The model under review builds one solid part; all positions refer to its coordinate system, in mm. A direction names the side the tool comes from. Coordinates: 2 decimals unless noted, no trailing zeros. Loops run counter-clockwise (first coordinate to the right, second up) from the corner with the lowest first, then second, coordinate; pieces in that order, holes last. Notation, with made-up numbers: (56, 89.5) - (95, 89.5) arc R29 cw to (95, 121.5) - close; hole circle Ø2 at (36.25, -20). An arc over 180 degrees is marked (long way). One line per item, written item: value. Start each with the question number.
1. We need section A-A, the plane z = 0. Give the boundary of the cut face in (x, y).
2. Insertion check: P1, Ø3, axis at x = -20.5, z = -4, coming from the -Y side; P2, Ø6, axis at y = 10.5, z = 4.5, coming from the -X side; P3, Ø6, axis at y = 10.5, z = -16.5, coming from the -X side. Each pin has a flat end and moves straight along its axis. Give the tip position at first contact, or say it passes through.
3. To check wall thickness, follow line 1 (X direction, y = 0.75, z = 0); line 2 (X direction, y = 14.25, z = -2); line 3 (Y direction, x = 18, z = -3). State the ranges of each line that lie inside material, in increasing order.
4. We need section B-B, the plane x = 0. Give the boundary of the cut face in (y, z).
5. Mouldability with a two-part tool opening along Z and no side actions: class faces 4 (the face through (-15.821, 7.395, -20.633)), 5 (the face through (-11, 14, 11)), 6 (the face through (11.5, 0, -5.3)) as +Z half, -Z half, draft (parallel to the pull), parting line (faces both ways), or undercut.
6. For faces 1 (the face through (-7.36, 0.51, 23.37)), 2 (the face through (7.36, 14.51, 23.37)), 3 (the face through (17.5, 15, -17.5)), list the 3-axis set-ups (+Z, -Z, +X, -X, +Y, -Y) from which the entire face can be reached by the end or side of a thin tool; tool diameter is ignored.
7. We need section C-C, the plane y = 3.5. Give the boundary of the cut face in (x, z).
8. We need section D-D, the plane z = 19. Give the boundary of the cut face in (x, y).
from build123d import *

# Parameters (mm, degrees)
CROQUIS1_R              = 26
CROQUIS1_R_2            = 12.5
SALIENTE_EXTRUIR1_DEPTH = 15
CROQUIS2_R              = 24.5
CROQUIS2_R_2            = 14
CORTAR_EXTRUIR1_DEPTH   = 1
CORTAR_EXTRUIR3_START   = -1
CROQUIS3_R              = 24.5
CROQUIS3_R_2            = 14
CORTAR_EXTRUIR3_DEPTH   = 1


with BuildPart() as part:
    # Croquis1 → Saliente-Extruir1 (new body)
    with BuildSketch(Plane(origin=(0, 0, 0), x_dir=(1, 0, 0), z_dir=(0, 1, 0))):
        with Locations(Location((0, 0, 0), (0, 0, 270))):
            Circle(CROQUIS1_R)
        with Locations(Location((0, 0, 0), (0, 0, 270))):
            Circle(CROQUIS1_R_2, mode=Mode.SUBTRACT)
    extrude(amount=SALIENTE_EXTRUIR1_DEPTH)

    # Croquis2 → Cortar-Extruir1 (cut)
    with BuildSketch(Plane(origin=(0, 15, 0), x_dir=(1, 0, 0), z_dir=(0, 1, 0))):
        with Locations(Location((0, 0, 0), (0, 0, 270))):
            Circle(CROQUIS2_R)
        with Locations(Location((0, 0, 0), (0, 0, 270))):
            Circle(CROQUIS2_R_2, mode=Mode.SUBTRACT)
    extrude(amount=-CORTAR_EXTRUIR1_DEPTH, mode=Mode.SUBTRACT)

    # Croquis3 → Cortar-Extruir3 (cut)
    with BuildSketch(Plane.XZ.offset(CORTAR_EXTRUIR3_START)):
        with Locations(Location((0, 0, 0), (0, 0, 90))):
            Circle(CROQUIS3_R)
        with Locations(Location((0, 0, 0), (0, 0, 90))):
            Circle(CROQUIS3_R_2, mode=Mode.SUBTRACT)
    extrude(amount=CORTAR_EXTRUIR3_DEPTH, mode=Mode.SUBTRACT)


solid = part.part
Findings below:
1. outline: (-26, 0) - (-24.5, 0) - (-24.5, 1) - (-14, 1) - (-14, 0) - (-12.5, 0) - (-12.5, 15) - (-14, 15) - (-14, 14) - (-24.5, 14) - (-24.5, 15) - (-26, 15) - close; (12.5, 0) - (14, 0) - (14, 1) - (24.5, 1) - (24.5, 0) - (26, 0) - (26, 15) - (24.5, 15) - (24.5, 14) - (14, 14) - (14, 15) - (12.5, 15) - close
2. P1: y = 1
2. P2: x = -25.96
2. P3: x = -22.22
3. line 1: -26 to -24.5, -14 to -12.5, 12.5 to 14, 24.5 to 26
3. line 2: -25.92 to -24.42, -13.86 to -12.34, 12.34 to 13.86, 24.42 to 25.92
3. line 3: 1 to 14
4. outline: (0, -26) - (15, -26) - (15, -24.5) - (14, -24.5) - (14, -14) - (15, -14) - (15, -12.5) - (0, -12.5) - (0, -14) - (1, -14) - (1, -24.5) - (0, -24.5) - close; (0, 12.5) - (15, 12.5) - (15, 14) - (14, 14) - (14, 24.5) - (15, 24.5) - (15, 26) - (0, 26) - (0, 24.5) - (1, 24.5) - (1, 14) - (0, 14) - close
5. face 4: parting line
5. face 5: undercut
5. face 6: draft
6. face 1: -Y
6. face 2: +Y
6. face 3: +Z, -Z, +X, -X, +Y
7. outline: circle Ø52 at (0, 0); hole circle Ø25 at (0, 0)
8. outline: (-17.75, 0) - (-15.47, 0) - (-15.47, 1) - (15.47, 1) - (15.47, 0) - (17.75, 0) - (17.75, 15) - (15.47, 15) - (15.47, 14) - (-15.47, 14) - (-15.47, 15) - (-17.75, 15) - close
